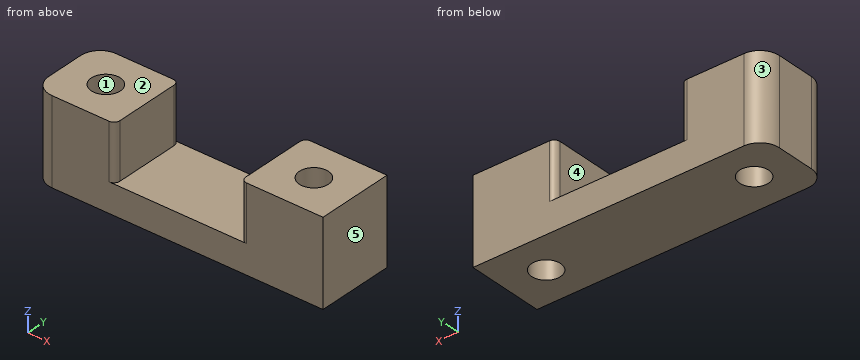
Autodesk Inventor part; units mm, degrees
ref_plane "YZ Plane" through (0, 0, 0) normal (1, 0, 0) x (0, 1, 0)
ref_plane "XZ Plane" through (0, 0, 0) normal (0, 1, 0) x (-1, 0, 0)
ref_plane "XY Plane" through (0, 0, 0) normal (0, 0, 1) x (1, 0, 0)
sketch "Sketch1" plane through (0, 0, 0) normal (0, 0, 1) x (1, 0, 0)
  line L0 (-2.4507, 4.6791) -> (10.5493, 4.6791)
  line L1 (10.5493, 4.6791) -> (10.5493, -3.3209)
  line L2 (10.5493, -3.3209) -> (-2.4507, -3.3209)
  line L3 (-2.4507, -3.3209) -> (-2.4507, 4.6791)
  line L4 (-2.4507, 4.6791) -> (-10.9507, 4.6791)
  line L5 (-10.9507, 4.6791) -> (-10.9507, -3.3209)
  line L6 (-10.9507, -3.3209) -> (-2.4507, -3.3209)
  line L7 (10.5493, -3.3209) -> (19.0493, -3.3209)
  line L8 (19.0493, -3.3209) -> (19.0493, 4.6791)
  line L9 (19.0493, 4.6791) -> (10.5493, 4.6791)
  point P0 (0, 0)
  point P1 (-6.7007, 0.6791)
  point P2 (14.7993, 0.6791)
  dimension "d0" = 13
  dimension "d1" = 8
  dimension "d2" = 8.5
  dimension "d3" = 8.5
  dimension "d4" = 30
  dimension "d5" = 4.25
  dimension "d6" = 4
  dimension "d7" = 4
  dimension "d8" = 4.25
extrude "Extrusion1" add sketch "Sketch1" along normal blind 5.75 contours L3 L6 L5 L4 | L9 L8 L7 L1
extrude "Extrusion2" add sketch "Sketch1" against normal blind 3
hole "Hole1" at (-6.7007, 0.6791, 0) at (14.7993, 0.6791, 0) direction (0, 0, 1) diameter 3 end through all both
fillet "Fillet1" radius 2 2 edges at (-10.9507, -3.3209, 1.375) (-10.9507, 4.6791, 1.375)
fillet "Fillet2" radius 0.6 4 edges at (10.5493, -3.3209, 2.875) (-2.4507, -3.3209, 2.875) (10.5493, 4.6791, 2.875) (-2.4507, 4.6791, 2.875)
equation "\"d3\" = d2"
properties part number "3DP_PLA_Y_axis_endstop_mount" material "ABS Plastic"
Here's how the part is built. I have some questions about the finished solid (model axes, mm). Face numbers are marked on the shaded views. A direction names the side the tool comes from. Give positions to 0.01 mm unless a question says otherwise; leave off trailing zeros. Loops run counter-clockwise (first coordinate to the right, second up) from the corner with the lowest first, then second, coordinate; pieces in that order, holes last. Notation, with made-up numbers: M -9,-11 L 11,-11 A24 ccw 11,1 Z; hole C -15,-2 d10. An arc over 180 degrees is marked long. Put each result on its own line as item: value. Start each with the question number.
(1) For the marked faces 4 and 5, which set-ups out of +Z, -Z, +X, -X, +Y, -Y let a thin tool reach every point of the face, with its end or its side?
(2) Will these pins go through, and if not, where does the flat tip stop? pin 1 Ø3 at (x, y) = (4.5, 1.5) entering from +Z; pin 2 Ø2.5 at (x, y) = (14.8, 0.68) entering from -Z.
(3) I want a section at D-D on z = -1. Please give me the cut outline in (x, y).
(4) I want a section at B-B on z = 2. Please give me the cut outline in (x, y), then the cut area to 3 significant figures.
(5) I want a section at A-A on x = -6.25. Please give me the cut outline in (y, z).
(6) I want a section at C-C on y = 1.5. Please give me the cut outline in (x, z), then the cut area to 3 significant figures.
(7) If we mould it in two halves opening along Y, with no side actions, what happens to the marked faces 1, 2 and 3? For each: +Y half, -Y half, draft (parallel to the pull), parting line (faces both ways), or undercut.
(8) I need wall thicknesses on line 1 along X through (y, z) = (2.5, 3); line 2 along Z through (x, y) = (-1, 2); line 3 along Y through (x, z) = (-6, 2.25). Which ranges of each line are inside material? Lowest first, please. Write a range as [from, to].
Answer block:
1. face 4: +Z, +Y, -Y
1. face 5: +Z, -Z, +X, +Y, -Y
2. pin 1: z = 0
2. pin 2: through
3. outline: M -10.95,-1.32 A2 ccw -8.95,-3.32 L 19.05,-3.32 L 19.05,4.68 L -8.95,4.68 A2 ccw -10.95,2.68 Z; hole C -6.7,0.68 d3; hole C 14.8,0.68 d3
4. outline: M -10.95,-1.32 A2 ccw -8.95,-3.32 L -3.05,-3.32 A0.6 ccw -2.45,-2.72 L -2.45,4.08 A0.6 ccw -3.05,4.68 L -8.95,4.68 A2 ccw -10.95,2.68 Z; M 10.55,-2.72 A0.6 ccw 11.15,-3.32 L 19.05,-3.32 L 19.05,4.68 L 11.15,4.68 A0.6 ccw 10.55,4.08 Z; hole C -6.7,0.68 d3; hole C 14.8,0.68 d3
4. area: 120 mm^2
5. outline: M -3.32,-3 L -0.75,-3 L -0.75,5.75 L -3.32,5.75 Z; M 2.11,-3 L 4.68,-3 L 4.68,5.75 L 2.11,5.75 Z
6. outline: M -10.95,-3 L -7.96,-3 L -7.96,5.75 L -10.95,5.75 Z; M -5.45,-3 L 13.54,-3 L 13.54,5.75 L 10.55,5.75 L 10.55,0 L -2.45,0 L -2.45,5.75 L -5.45,5.75 Z; M 16.05,-3 L 19.05,-3 L 19.05,5.75 L 16.05,5.75 Z
6. area: 144 mm^2
7. face 1: undercut
7. face 2: draft
7. face 3: +Y half
8. line 1: [-10.95, -2.45], [10.55, 19.05]
8. line 2: [-3, 0]
8. line 3: [-3.32, -0.65], [2.01, 4.68]
